Geometry check sheet. Reference: the model listing, model coordinates, mm. Coordinates: 2 decimals unless noted, no trailing zeros. Loops run counter-clockwise (first coordinate to the right, second up) from the corner with the lowest first, then second, coordinate; pieces in that order, holes last.
from build123d import *

# Parameters (mm, degrees)
SKETCH1_W           = 400
SKETCH1_H           = 350
SKETCH1_R           = 1.5
BOSS_EXTRUDE1_DEPTH = 4
CUT_EXTRUDE1_DEPTH  = 10


with BuildPart() as part:
    # Sketch1 → Boss-Extrude1 (new body)
    with BuildSketch(Plane.XY):
        Rectangle(SKETCH1_W, SKETCH1_H)
        with Locations((190.420210886, -135)):
            Circle(SKETCH1_R, mode=Mode.SUBTRACT)
        with Locations((190.420210886, -115)):
            Circle(SKETCH1_R, mode=Mode.SUBTRACT)
        with Locations((190.420210886, -95)):
            Circle(SKETCH1_R, mode=Mode.SUBTRACT)
        with Locations((190, 68.62)):
            Circle(SKETCH1_R, mode=Mode.SUBTRACT)
        with Locations((190, 88.62)):
            Circle(SKETCH1_R, mode=Mode.SUBTRACT)
        with Locations((190, 108.62)):
            Circle(SKETCH1_R, mode=Mode.SUBTRACT)
        with Locations(Location((-190.420210886, -135, 0), (0, 0, 180))):
            Circle(SKETCH1_R, mode=Mode.SUBTRACT)
        with Locations(Location((-190.420210886, -95, 0), (0, 0, 180))):
            Circle(SKETCH1_R, mode=Mode.SUBTRACT)
        with Locations(Location((-190.420210886, -115, 0), (0, 0, 180))):
            Circle(SKETCH1_R, mode=Mode.SUBTRACT)
        with Locations(Location((-190, 68.62, 0), (0, 0, 180))):
            Circle(SKETCH1_R, mode=Mode.SUBTRACT)
        with Locations(Location((-190, 88.62, 0), (0, 0, 180))):
            Circle(SKETCH1_R, mode=Mode.SUBTRACT)
        with Locations(Location((-190, 108.62, 0), (0, 0, 180))):
            Circle(SKETCH1_R, mode=Mode.SUBTRACT)
    extrude(amount=BOSS_EXTRUDE1_DEPTH)

    # Sketch2 → Cut-Extrude1 (cut)
    with BuildSketch(Plane.XY.offset(4)):
        Polygon((-76.924392285, 70.222779709), (-156.531783107, 6.536867051), (-143.98758819, 30.17784978), (-64.380197367, 93.863762438), align=None)
        Polygon((15.0683317, 118.246100027), (-64.539059123, 54.560187369), (-51.994864205, 78.201170098), (27.612526617, 141.887082756), align=None)
        Polygon((20.075418883, 76.706692842), (-59.53197194, 13.020780184), (-46.987777022, 36.661762913), (32.6196138, 100.347675571), align=None)
        Polygon((112.068142867, 124.730013159), (32.460752045, 61.044100501), (45.004946962, 84.685083231), (124.612337785, 148.370995889), align=None)
        Polygon((163.398141207, 99.888741611), (83.790750385, 36.202828953), (57.972773228, 29.154074023), (137.580164051, 92.839986681), align=None)
        Polygon((5.854349879, 13.609157056), (-73.753040943, -50.076755602), (-61.208846026, -26.435772873), (18.398544797, 37.250139785), align=None)
        Polygon((31.672327036, 20.657911987), (-47.935063786, -43.028000671), (-73.753040943, -50.076755602), (5.854349879, 13.609157056), align=None)
        Polygon((135.779730821, 6.678077501), (56.172339999, -57.007835157), (30.354362842, -64.056590088), (109.961753665, -0.37067743), align=None)
        Polygon((68.734186222, -72.529217049), (-10.8732046, -136.215129707), (-36.691181757, -143.263884637), (42.916209066, -79.577971979), align=None)
        Polygon((-91.145461288, 7.125243924), (-170.752852111, -56.560668734), (-158.208657193, -32.919686005), (-78.601266371, 30.766226653), align=None)
        Polygon((70.534619452, 13.632692131), (-9.072771371, -50.053220527), (16.745205786, -43.004465597), (96.352596608, 20.681447061), align=None)
        Polygon((-21.764060506, -79.601507054), (-101.371451329, -143.287419712), (-75.553474172, -136.238664782), (4.05391665, -72.552752124), align=None)
        Polygon((-85.129533688, -56.876544129), (-152.460215151, -113.62145781), (-164.039471998, -136.238664782), (-96.708790535, -79.493751101), align=None)
    extrude(amount=-CUT_EXTRUDE1_DEPTH, mode=Mode.SUBTRACT)


solid = part.part
1) Material ranges on probe 1 along X at (y, z) = (-95, 1.75); probe 2 along X at (y, z) = (-51, 2.95); probe 3 along Y at (x, z) = (-127.5, 0.4), recorded low to high.
Data:
probe 1: x = -200 to -191.92, -188.92 to -130.36, -115.11 to -41.01, -24.01 to 23.64, 40.65 to 188.92, 191.92 to 200
probe 2: x = -200 to -167.8, -163.8 to 46.68, 63.68 to 200
probe 3: y = -175 to -105.44, -92.59 to -21.96, -8.35 to 29.76, 43.37 to 175
2) Mould release check, pull along Y, two halves, no side actions. Record for faces 1 (the flat face through (31.288, -17.764, 2.028)), 2 (the flat face through (-24.178, 86.849, 2.028)): +Y half, -Y half, draft (parallel to the pull), parting line (faces both ways), or undercut.
Data:
face 1: undercut
face 2: undercut
3) Section check B-B on z = 1.9. Count the separate pieces of the cut face and the enclosed holes in it, and give its area (3 significant figures).
Data:
separate pieces: 1
enclosed holes: 24
area: 126,000 mm2
4) Section check A-A on y = -127. Record the cut outline in (x, z), and give its area (3 significant figures).
Data:
outline: (-200, 0) - (-159.31, 0) - (-159.31, 4) - (-200, 4) - close; (-153.08, 0) - (-81.01, 0) - (-81.01, 4) - (-153.08, 4) - close; (-64.01, 0) - (-16.36, 0) - (-16.36, 4) - (-64.01, 4) - close; (0.65, 0) - (200, 0) - (200, 4) - (0.65, 4) - close
area: 1,440 mm2
